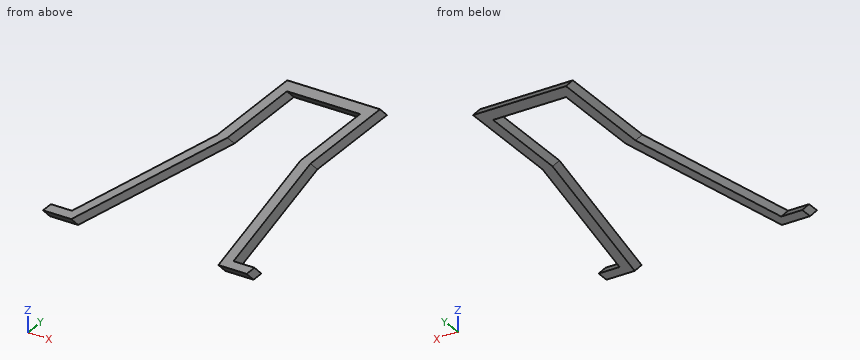
from build123d import *


with BuildPart() as f2:
    # F2: sweep along a path in F1
    with BuildLine(Plane.YZ) as f2_path:
        Line((0, 0), (-5.2465468888, 5.2465468888))
    # F0 (on Top) → F2 (sweep)
    with BuildSketch(Plane.XY):
        Polygon((-17.5813417882, -13.8564798981), (-17.5813417882, 31.3983540978), (17.5813417882, 31.3983540978), (17.5813417882, -13.8564798981), (35.3969819844, -104.5009791851), (38.8697721064, -104.5009791851), (48.9724315703, -104.5009791851), (48.9724315703, -98.5025316477), (38.8697721064, -98.5025316477), (22.3438417882, -13.8564798981), (22.3438417882, 39.0965069434), (0, 39.0965069434), (-22.3438417882, 39.0965069434), (-22.3438417882, -13.8564798981), (-38.8697721064, -98.5025316477), (-48.9724315703, -98.5025316477), (-48.9724315703, -104.5009791851), (-38.8697721064, -104.5009791851), (-35.3969819844, -104.5009791851), align=None)
    sweep(path=f2_path.line)


solid = f2.part
Verification items for the finished model (mm, model axes). Give positions to 0.01 mm unless a question says otherwise; leave off trailing zeros. Loops run counter-clockwise (first coordinate to the right, second up) from the corner with the lowest first, then second, coordinate; pieces in that order, holes last.
1. Cross-section at B-B on y = -74. Record the cut outline in (x, z), and give its area (3 significant figures).
Derived:
outline: (-34.09, 0) - (-29.4, 0) - (-28.37, 5.25) - (-33.06, 5.25) - close; (28.37, 5.25) - (29.4, 0) - (34.09, 0) - (33.06, 5.25) - close
area: 49.2 mm2
2. Cross-section at D-D on x = 13. Record the cut outline in (y, z), and give its area (3 significant figures).
Derived:
outline: (26.15, 5.25) - (31.4, 0) - (39.1, 0) - (33.85, 5.25) - close
area: 40.4 mm2
3. Cross-section at C-C on z = 4.1. Record the cut outline in (x, y), and give its area (3 significant figures).
Derived:
outline: (-48.97, -108.6) - (-35.4, -108.6) - (-17.58, -17.96) - (-17.58, 27.3) - (17.58, 27.3) - (17.58, -17.96) - (35.4, -108.6) - (48.97, -108.6) - (48.97, -102.6) - (38.87, -102.6) - (22.34, -17.96) - (22.34, 35) - (-22.34, 35) - (-22.34, -17.96) - (-38.87, -102.6) - (-48.97, -102.6) - close
area: 1,740 mm2
4. Go/stop test with flat-tipped pins: P1, Ø1, axis at y = -47.5, z = 2, coming from the +X side; P2, Ø1.6, axis at y = 7, z = 1.5, coming from the -X side; P3, Ø1.6, axis at y = 22.5, z = 3.5, coming from the +X side. Record where each tip stops, or that it passes through.
Derived:
P1: stops at x = 28.66
P2: stops at x = -22.34
P3: stops at x = 22.34
5. Cross-section at A-A on y = -2.5. Record the cut outline in (x, z), and give its area (3 significant figures).
Derived:
outline: (-22.34, 0) - (-17.58, 0) - (-17.58, 5.25) - (-22.34, 5.25) - close; (17.58, 0) - (22.34, 0) - (22.34, 5.25) - (17.58, 5.25) - close
area: 50.0 mm2
6. Material ranges on probe 1 along X at (y, z) = (14, 1.8); probe 2 along X at (y, z) = (30, 3.75); probe 3 along X at (y, z) = (-22.5, 1.8), recorded low to high.
Derived:
probe 1: x = -22.34 to -17.58, 17.58 to 22.34
probe 2: x = -22.34 to 22.34
probe 3: x = -23.68 to -18.93, 18.93 to 23.68
